Can you work these out from the model? Positions are in its coordinate system, mm. A direction names the side the tool comes from. Give positions to 0.01 mm unless a question says otherwise; leave off trailing zeros. Loops run counter-clockwise (first coordinate to the right, second up) from the corner with the lowest first, then second, coordinate; pieces in that order, holes last. Notation, with made-up numbers: (-5.75, 41) -> (19.25, 41) arc R6 cw to (19.25, 52) -> close; hole circle Ø3 at (49, 43.5). An arc over 180 degrees is marked (long way). One line per question, with ' | ' between items.
Autodesk Inventor part; units mm, degrees
ref_plane "YZ Plane" through (0, 0, 0) normal (1, 0, 0) x (0, 1, 0)
ref_plane "XZ Plane" through (0, 0, 0) normal (0, 1, 0) x (-1, 0, 0)
ref_plane "XY Plane" through (0, 0, 0) normal (0, 0, 1) x (1, 0, 0)
sketch "Sketch1" plane through (0, 0, 0) normal (1, 0, 0) x (0, 1, 0)
  line L0 (41, 19.75) -> (-41, 19.75)
  line L1 (-41, 19.75) -> (-41, -19.75)
  line L2 (-41, -19.75) -> (41, -19.75)
  line L3 (41, -19.75) -> (41, 19.75)
  line L4 (41, 19.75) -> (-41, -19.75) construction
  line L5 (-41, 19.75) -> (41, -19.75) construction
  circle A0 centre (19.75, 0) radius 12.5
  line L6 (35.2464, 15.4749) -> (32.7715, 13) construction
  line L7 (34.1504, 16.5709) -> (31.6755, 14.096)
  line L8 (33.8675, 11.904) -> (36.3424, 14.3789)
  arc A1 (36.3424, 14.3789) -> (34.1504, 16.5709) centre (35.2464, 15.4749) ccw
  arc A2 (31.6755, 14.096) -> (33.8675, 11.904) centre (32.7715, 13) ccw
  line L9 (35.2464, -15.4749) -> (32.7715, -13) construction
  line L10 (36.3424, -14.3789) -> (33.8675, -11.904)
  line L11 (31.6755, -14.096) -> (34.1504, -16.5709)
  arc A3 (34.1504, -16.5709) -> (36.3424, -14.3789) centre (35.2464, -15.4749) ccw
  arc A4 (33.8675, -11.904) -> (31.6755, -14.096) centre (32.7715, -13) ccw
  line L12 (6.7715, -13) -> (4.2966, -15.4749) construction
  line L13 (5.6755, -11.904) -> (3.2006, -14.3789)
  line L14 (5.3927, -16.5709) -> (7.8675, -14.096)
  arc A5 (7.8675, -14.096) -> (5.6755, -11.904) centre (6.7715, -13) ccw
  arc A6 (3.2006, -14.3789) -> (5.3927, -16.5709) centre (4.2966, -15.4749) ccw
  line L15 (6.7715, 13) -> (4.2966, 15.4749) construction
  line L16 (7.8675, 14.096) -> (5.3927, 16.5709)
  line L17 (3.2006, 14.3789) -> (5.6755, 11.904)
  arc A7 (5.6755, 11.904) -> (7.8675, 14.096) centre (6.7715, 13) ccw
  arc A8 (5.3927, 16.5709) -> (3.2006, 14.3789) centre (4.2966, 15.4749) ccw
  line L18 (-57.4, 0) -> (57.4, 0) construction
  line L19 (0, -27.65) -> (0, 27.65) construction
  circle A9 centre (-32.8, 10) radius 2.55
  circle A10 centre (-32.8, 0) radius 2.55
  circle A11 centre (-32.8, -10) radius 2.55
  circle A12 centre (-12.8, 10) radius 2.55
  circle A13 centre (-12.8, -10) radius 2.55
  circle A14 centre (-12.8, 0) radius 2.55
  point P0 (0, 0)
  point P1 (34.009, 14.2374)
  point P2 (34.009, -14.2374)
  point P3 (5.5341, -14.2374)
  point P4 (5.5341, 14.2374)
  dimension "d0" = 82
  dimension "d1" = 39.5
  dimension "d2" = 25
  dimension "d3" = 21.25
  dimension "d4" = 45
  dimension "d5" = 45
  dimension "d6" = 45
  dimension "d7" = 3.5
  dimension "d8" = 3.5
  dimension "d9" = 3.5
  dimension "d10" = 3.5
  dimension "d11" = 3.1
  dimension "d12" = 3.1
  dimension "d13" = 3.1
  dimension "d14" = 3.1
  dimension "d16" = 18.4
  dimension "d17" = 26
  dimension "d19" = 26
  dimension "d20" = 13
  dimension "d21" = 5.1
  dimension "d22" = 5.1
  dimension "d23" = 5.1
  dimension "d24" = 5.1
  dimension "d25" = 5.1
  dimension "d26" = 5.1
  dimension "d27" = 8.2
  dimension "d28" = 9.75
  dimension "d29" = 9.75
  dimension "d30" = 20
extrude "Plate1" add sketch "Sketch1" along normal mid plane 3
fillet "Corner Round1" radius 6 4 edges at (0, 41, 19.75) (0, 41, -19.75) (0, -41, 19.75) (0, -41, -19.75)
equation "\"d8\" = d7"
equation "\"d22\" = d21"
equation "\"d23\" = d22"
equation "\"d24\" = d23"
equation "\"d25\" = d24"
equation "\"d26\" = d24"
equation "\"d31\" = Thickness"
equation "\"BendRadius\" = Thickness"
equation "\"BendReliefWidth\" = Thickness"
equation "\"BendReliefDepth\" = 0.5 * Thickness"
equation "\"CornerReliefSize\" = 4 * Thickness"
equation "\"MinimumRemnant\" = 2 * Thickness"
equation "\"TransitionRadius\" = BendRadius"
equation "\"JacobiRadiusSize\" = BendRadius"
equation "\"GapSize\" = Thickness"
properties part number "HCMUTE-CDT23-OP_GA-STEP-42"
Q1. If we section it at A-A (z = 0): Write out the boundary of the cut face in (x, y), plus the area to 3 significant figures.
Entries:
outline: (-1.5, -41) -> (1.5, -41) -> (1.5, -35.35) -> (-1.5, -35.35) -> close; (-1.5, -30.25) -> (1.5, -30.25) -> (1.5, -15.35) -> (-1.5, -15.35) -> close; (-1.5, -10.25) -> (1.5, -10.25) -> (1.5, 7.25) -> (-1.5, 7.25) -> close; (-1.5, 32.25) -> (1.5, 32.25) -> (1.5, 41) -> (-1.5, 41) -> close | area: 140 mm²
Q2. If we mould it in two halves opening along Z, with no side actions, what happens to faces 3 (the face through (0.021, -39.196, 18.039)), 4 (the face through (-0.021, -35.348, -0.112)), 5 (the face through (-1.5, -1, 0)), 6 (the face through (-0.021, 36.366, -16.547))? For each: pulls with the +Z half, pulls with the -Z half, needs draft (parallel to the pull), parting line crosses it, or undercut.
Entries:
face 3: pulls with the +Z half | face 4: undercut | face 5: needs draft | face 6: undercut
Q3. If I drill on probe 1 along Z at (x, y) = (0.85, -12.8); probe 2 along Y at (x, z) = (1.3, -8); probe 3 along Z at (x, y) = (0.5, 19.75), over which ranges is the centre line in solid material (lowest first)? Write a range as from..to.
Entries:
probe 1: -19.75..-12.55, -7.45..-2.55, 2.55..7.45, 12.55..19.75 | probe 2: -41..-34.38, -31.22..-14.38, -11.22..10.15, 29.35..41 | probe 3: -19.75..-12.5, 12.5..19.75
Q4. If we section it at D-D (y = -32.8): Write out the boundary of the cut face in (x, z).
Entries:
outline: (-1.5, -19.75) -> (1.5, -19.75) -> (1.5, -12.55) -> (-1.5, -12.55) -> close; (-1.5, -7.45) -> (1.5, -7.45) -> (1.5, -2.55) -> (-1.5, -2.55) -> close; (-1.5, 2.55) -> (1.5, 2.55) -> (1.5, 7.45) -> (-1.5, 7.45) -> close; (-1.5, 12.55) -> (1.5, 12.55) -> (1.5, 19.75) -> (-1.5, 19.75) -> close
Q5. For pin 1 Ø4.5 at (y, z) = (-12.8, -10) entering from -X; pin 2 Ø6.5 at (y, z) = (-12.8, 0) entering from +X, each with a flat end and sliding along its axis, tell me the tip position at first contact or that it passes through.
Entries:
pin 1: through | pin 2: x = 1.5
Q6. On a 3-axis mill with a long thin cutter (end or side, diameter ignored), from which of +Z, -Z, +X, -X, +Y, -Y can I reach the whole of each face in a straight line? I mean faces 1 (the face through (0, 41, 0)), 2 (the face through (-0.02, 32.9, -15.32)). Say none if no direction works.
Entries:
face 1: +Z, -Z, +X, -X, +Y | face 2: +X, -X
Q7. If we section it at C-C (x = -0.85): State how many separate pieces and enclosed holes the cut face has, plus the area to 3 significant figures.
Entries:
separate pieces: 1 | enclosed holes: 11 | area: 2,520 mm²
Q8. If we section it at B-B (y = 19.75): Write out the boundary of the cut face in (x, z), plus the area to 3 significant figures.
Entries:
outline: (-1.5, -19.75) -> (1.5, -19.75) -> (1.5, -12.5) -> (-1.5, -12.5) -> close; (-1.5, 12.5) -> (1.5, 12.5) -> (1.5, 19.75) -> (-1.5, 19.75) -> close | area: 43.5 mm²
